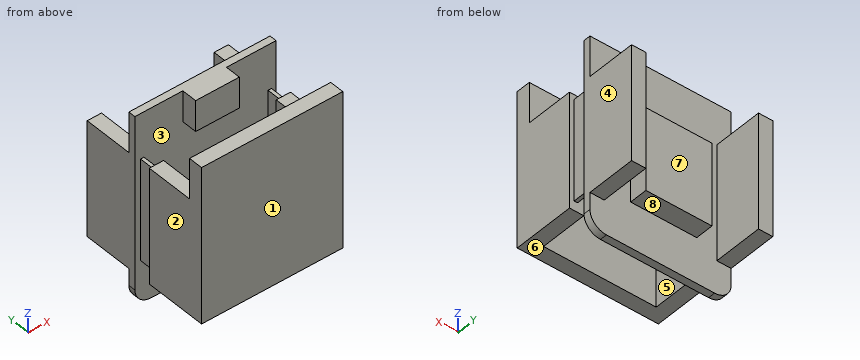
Autodesk Inventor part; units mm, degrees
ref_plane "YZ Plane" through (0, 0, 0) normal (1, 0, 0) x (0, 1, 0)
ref_plane "XZ Plane" through (0, 0, 0) normal (0, 1, 0) x (-1, 0, 0)
ref_plane "XY Plane" through (0, 0, 0) normal (0, 0, 1) x (1, 0, 0)
sketch "Sketch1" plane through (0, 0, 0) normal (0, 1, 0) x (-1, 0, 0)
  line L0 (2.4457, 9.8333) -> (-23.1743, 9.8333)
  line L1 (-23.1743, 9.8333) -> (-23.1743, -18.5067)
  line L2 (-23.1743, -18.5067) -> (2.4457, -18.5067)
  line L3 (2.4457, -18.5067) -> (2.4457, 9.8333)
  point P0 (0, 0)
  dimension "d0" = 28.34
  dimension "d1" = 25.62
extrude "Extrusion1" add sketch "Sketch1" along normal blind 2.6
sketch "Sketch2" plane through (0, 2.6, 0) normal (0, 1, 0) x (1, 0, 0)
  line L0 (23.1743, 18.5067) -> (-2.4457, 18.5067)
  line L1 (-2.4457, 18.5067) -> (0.1443, 18.5067)
  line L2 (0.1443, 18.5067) -> (0.1443, -2.4933)
  line L3 (0.1443, -2.4933) -> (-2.4457, -2.4933)
  line L4 (-2.4457, -2.4933) -> (-2.4457, 18.5067)
  point P0 (0, 0)
  dimension "d4" = 21
  dimension "d5" = 2.59
extrude "Extrusion2" add sketch "Sketch2" along normal blind 8.7
sketch "Sketch3" plane through (0, 2.6, 0) normal (0, 1, 0) x (1, 0, 0)
  line L0 (23.1743, 18.5067) -> (20.5843, 18.5067)
  line L1 (20.5843, 18.5067) -> (20.5843, -2.4933)
  line L2 (20.5843, -2.4933) -> (23.1743, -2.4933)
  line L3 (23.1743, -2.4933) -> (23.1743, 18.5067)
  point P0 (0, 0)
  dimension "d8" = 21
  dimension "d9" = 2.59
extrude "Extrusion3" add sketch "Sketch3" along normal blind 8.7
sketch "Sketch4" plane through (0, 11.3, 0) normal (0, 1, 0) x (1, 0, 0)
  line L0 (-1.4241, 16.7919) -> (-0.8041, 16.7919)
  line L1 (-0.8041, 16.7919) -> (-0.8041, -1.6081)
  line L2 (-0.8041, -1.6081) -> (-1.4241, -1.6081)
  line L3 (-1.4241, -1.6081) -> (-1.4241, 16.7919)
  line L4 (21.7236, 16.7919) -> (22.3436, 16.7919)
  line L5 (22.3436, 16.7919) -> (22.3436, -1.6081)
  line L6 (22.3436, -1.6081) -> (21.7236, -1.6081)
  line L7 (21.7236, -1.6081) -> (21.7236, 16.7919)
  point P0 (0, 0)
  dimension "d14" = 18.4
  dimension "d15" = 0.62
  dimension "d16" = 18.4
  dimension "d17" = 0.62
extrude "Extrusion4" add sketch "Sketch4" along normal blind 3.12
sketch "Sketch5" plane through (0, 14.42, 0) normal (0, 1, 0) x (1, 0, 0)
  line L0 (-2.4457, -9.8333) -> (23.1743, -9.8333)
  line L1 (23.1743, -9.8333) -> (23.1743, -2.4933)
  line L2 (-2.4457, -9.8333) -> (23.1743, -9.8333)
  line L3 (23.1743, -9.8333) -> (23.1743, 21.5867)
  line L4 (20.1743, 24.5867) -> (0.5543, 24.5867)
  line L5 (-2.4457, 21.5867) -> (-2.4457, -9.8333)
  arc A0 (0.5543, 24.5867) -> (-2.4457, 21.5867) centre (0.5543, 21.5867) ccw
  arc A1 (23.1743, 21.5867) -> (20.1743, 24.5867) centre (20.1743, 21.5867) ccw
  point P0 (0, 0)
  point P1 (-2.4457, 24.5867)
  dimension "d18" = 34.42
  dimension "d19" = 3
extrude "Extrusion5" add sketch "Sketch5" along normal blind 1.3
sketch "Sketch6" plane through (0, 15.72, 0) normal (0, 1, 0) x (1, 0, 0)
  line L0 (-2.4457, -2.4933) -> (0.1443, -2.4933)
  line L1 (0.1443, 18.5067) -> (-2.4457, 18.5067)
  line L2 (-2.4457, -2.4933) -> (0.1443, -2.4933)
  line L3 (0.1443, -2.4933) -> (0.1443, 18.5067)
  line L4 (0.1443, 18.5067) -> (-2.4457, 18.5067)
  line L5 (-2.4457, 18.5067) -> (-2.4457, -2.4933)
  line L6 (23.1743, -2.4933) -> (20.5843, -2.4933)
  line L7 (20.5843, 18.5067) -> (0.1443, 18.5067)
  line L8 (23.1743, -2.4933) -> (20.5843, -2.4933)
  line L9 (20.5843, -2.4933) -> (20.5843, 18.5067)
  line L10 (20.5843, 18.5067) -> (23.1743, 18.5067)
  line L11 (23.1743, 18.5067) -> (23.1743, -2.4933)
  point P0 (0, 0)
extrude "Extrusion6" add sketch "Sketch6" along normal blind 9
sketch "Sketch7" plane through (0, 15.72, 0) normal (0, 1, 0) x (1, 0, 0)
  line L0 (3.7943, 16.2867) -> (15.7943, 16.2867)
  line L1 (15.7943, 16.2867) -> (15.7943, 1.2867)
  line L2 (15.7943, 1.2867) -> (3.7943, 1.2867)
  line L3 (3.7943, 1.2867) -> (3.7943, 16.2867)
  line L4 (20.5843, 18.5067) -> (20.5843, -2.4933)
  line L5 (-2.4457, -9.8333) -> (23.1743, -9.8333)
  point P0 (0, 0)
  dimension "d24" = 15
  dimension "d25" = 12
  dimension "d28" = 4.79
  dimension "d29" = 11.12
extrude "Extrusion7" add sketch "Sketch7" along normal blind 3.3
sketch "Sketch8" plane through (0, 14.42, 0) normal (0, -1, 0) x (1, 0, 0)
  line L0 (-2.4457, 9.8333) -> (23.1743, 9.8333)
  line L1 (14.1743, 9.8333) -> (6.2543, 9.8333)
  line L2 (6.2543, 9.8333) -> (6.2543, 4.2333)
  line L3 (6.2543, 4.2333) -> (14.1743, 4.2333)
  line L4 (14.1743, 4.2333) -> (14.1743, 9.8333)
  line L5 (23.1743, 9.8333) -> (23.1743, -21.5867)
  point P0 (0, 0)
  dimension "d30" = 9
  dimension "d31" = 7.92
  dimension "d32" = 5.6
extrude "Extrusion8" add sketch "Sketch8" along normal blind 2.78
equation "\"d16\" = d14"
equation "\"d17\" = d15"
properties part number "Wemos"
Check sheet for the modelled part. Datum: model origin and axes. Units: mm. Face numbers are marked on the shaded views. A direction names the side the tool comes from. Round coordinates to 2 decimals unless told otherwise and drop trailing zeros. Loops run counter-clockwise (first coordinate to the right, second up) from the corner with the lowest first, then second, coordinate; pieces in that order, holes last. Notation, with made-up numbers: (54, 37) -> (91, 37) arc R29 cw to (91, 58) -> close; hole circle Ø1 at (89.5, 16). An arc over 180 degrees is marked (long way). Put each result on its own line as item: value. Start each with the question number.
1. Section check B-B (x = 9.25). Enter the section's corners in (y, z), plus the area to 3 significant figures.
2. Section check D-D (y = 9.5). Enter the section's corners in (x, z).
3. Access from +Z, -Z, +X, -X, +Y, -Y to the whole of each face (thin tool, end or side, straight path). Record for the marked faces 5, 6, 7 and 8.
4. Section check A-A (z = 3). Enter the section's corners in (x, y), plus the area to 3 significant figures.
5. Scan lines: probe 1 along X at (y, z) = (17, -2); probe 2 along Y at (x, z) = (18.75, -3.5); probe 3 along Y at (x, z) = (20.75, 1). Record each from-to range of solid material in increasing order.
6. Draft check along X on the marked faces 1, 2, 3 and 4. Enter one of: +X half, -X half, draft (parallel to the pull), parting line (faces both ways), or undercut.
7. Section check C-C (y = 13.5). Enter the section's corners in (x, z), plus the area to 3 significant figures.
8. Gauge pin test, flat ends, axial feed: pin 1 (3.5 mm diameter, centred on x = 11.5, z = -7, fed in from +Y); pin 2 (0.5 mm diameter, centred on x = -1, y = 13, fed in from -Z); pin 3 (3 mm diameter, centred on x = 22, y = 7, fed in from +Z). Record the tip position at first contact, or that the pin passes through.
Findings:
1. outline: (0, -18.51) -> (2.6, -18.51) -> (2.6, 9.83) -> (0, 9.83) -> close; (11.64, 4.23) -> (14.42, 4.23) -> (14.42, -24.59) -> (15.72, -24.59) -> (15.72, -16.29) -> (19.02, -16.29) -> (19.02, -1.29) -> (15.72, -1.29) -> (15.72, 9.83) -> (11.64, 9.83) -> close
1. area: 183 mm^2
2. outline: (-2.45, -18.51) -> (0.14, -18.51) -> (0.14, 2.49) -> (-2.45, 2.49) -> close; (20.58, -18.51) -> (23.17, -18.51) -> (23.17, 2.49) -> (20.58, 2.49) -> close
3. face 5: +Z, -Z
3. face 6: -Z, +X, -X, -Y
3. face 7: +Z, -Z, +Y
3. face 8: -Z, +Y
4. outline: (-2.45, 0) -> (23.17, 0) -> (23.17, 2.6) -> (-2.45, 2.6) -> close; (-2.45, 14.42) -> (23.17, 14.42) -> (23.17, 15.72) -> (-2.45, 15.72) -> close
4. area: 99.9 mm^2
5. probe 1: x = -2.45 to 0.14, 3.79 to 15.79, 20.58 to 23.17
5. probe 2: y = 0 to 2.6, 14.42 to 15.72
5. probe 3: y = 0 to 11.3, 14.42 to 24.72
6. face 1: draft
6. face 2: -X half
6. face 3: undercut
6. face 4: +X half
7. outline: (-1.42, -16.79) -> (-0.8, -16.79) -> (-0.8, 1.61) -> (-1.42, 1.61) -> close; (6.25, 4.23) -> (14.17, 4.23) -> (14.17, 9.83) -> (6.25, 9.83) -> close; (21.72, -16.79) -> (22.34, -16.79) -> (22.34, 1.61) -> (21.72, 1.61) -> close
7. area: 67.2 mm^2
8. pin 1: stops at y = 19.02
8. pin 2: stops at z = -16.79
8. pin 3: stops at z = 2.49
